Can you work these out from the model? Positions are in its coordinate system, mm. A direction names the side the tool comes from. Coordinates: 2 decimals unless noted, no trailing zeros. Order: outer loops, then holes, each group sorted by start corner. A loop starts at its lowest first (then second) coordinate and runs counter-clockwise, first axis right, second up. Notation, with made-up numbers: (-5.5, 64.5) - (50.5, 64.5) arc R22 ccw to (50.5, 97.5) - close; hole circle Ø3 at (27, -5.75). An arc over 180 degrees is marked (long way). Return JSON: item names as keys, results as strings. Group by question number.
1) Which directions (+Z, -Z, +X, -X, +Y, -Y) give clear straight access to the entire face, cutting with the end or side of a thin tool? Please do faces 4 (the face through (12, -32, 11.049)), 5 (the face through (45, -13.005, 9)), 6 (the face through (16.002, -6, 18)).
2) Imagine slicing it at B-B (z = 23.5). Write out the boundary of the cut face in (x, y) (3 decimals).
3) Imagine slicing it at A-A (y = -6). Write out the boundary of the cut face in (x, z) (3 decimals), and give its area (3 significant figures).
4) Imagine slicing it at C-C (x = 6). Write out the boundary of the cut face in (y, z).
5) For pin 1 Ø5 at (x, z) = (33.5, 19.5) entering from +Y; pin 2 Ø4.5 at (x, y) = (7, -34) entering from +Z; pin 3 Ø18.5 at (y, z) = (-25.5, 5.5) entering from +X, each with a flat end and sliding along its axis, tell me the tip position at first contact or that it passes through.
6) If we mould it in two halves opening along X, with no side actions, what happens to faces 1 (the face through (48, 0, 18)), 2 (the face through (0, -14, 18)), 3 (the face through (28, -11.989, 18))? For each: pulls with the +X half, pulls with the -X half, needs draft (parallel to the pull), parting line crosses it, or undercut.
7) Imagine slicing it at D-D (y = -34.5). Write out the boundary of the cut face in (x, z).
8) If I drill on line 1 along X through (y, z) = (-7.5, 18) (3 decimals); line 2 along X through (y, z) = (-33.5, 25.5); line 3 along X through (y, z) = (-29.5, 7), over which ranges is the centre line in solid material (lowest first)?
```python
from build123d import *

# Parameters (mm, degrees)
F1_DEPTH = 35.9918
F2_W     = 24.9682
F2_H     = 8.9916
F3_DEPTH = 24.9428
F4_W     = 20.8534
F4_H     = 16.9418
F5_DEPTH = 24.003


with BuildPart() as f1:
    # F0 (on Top) → F1 (new body)
    with BuildSketch(Plane.XY):
        Polygon((16.002, 0), (0, 0), (0, -37.0078), (56.007, -37.0078), (56.007, 0), (40.005, 0), (40.005, -11.9888), (16.002, -11.9888), align=None)
    extrude(amount=F1_DEPTH)

    # F2 (on face) → F3 (cut)
    with BuildSketch(Plane.XY.offset(35.9918)):
        with Locations((12.4841, -32.512)):
            Rectangle(F2_W, F2_H)
    extrude(amount=-F3_DEPTH, mode=Mode.SUBTRACT)

    # F4 (on face) → F5 (cut)
    with BuildSketch(Plane.XZ.offset(37.0078)):
        with Locations((45.5803, 8.4709)):
            Rectangle(F4_W, F4_H)
    extrude(amount=-F5_DEPTH, mode=Mode.SUBTRACT)


solid = f1.part
```
Calculated:
{
 "1": {"face 4": "+Z, -X, -Y", "face 5": "-Z, +X, -Y", "face 6": "+Z, -Z, +Y"},
 "2": {"outline": "(0, -28.016) - (24.968, -28.016) - (24.968, -37.008) - (56.007, -37.008) - (56.007, 0) - (40.005, 0) - (40.005, -11.989) - (16.002, -11.989) - (16.002, 0) - (0, 0) - close"},
 "3": {"outline": "(0, 0) - (16.002, 0) - (16.002, 35.992) - (0, 35.992) - close; (40.005, 0) - (56.007, 0) - (56.007, 35.992) - (40.005, 35.992) - close", "area": "1,150 mm2"},
 "4": {"outline": "(-37.01, 0) - (0, 0) - (0, 35.99) - (-28.02, 35.99) - (-28.02, 11.05) - (-37.01, 11.05) - close"},
 "5": {"pin 1": "y = -11.99", "pin 2": "z = 11.05", "pin 3": "x = 35.15"},
 "6": {"face 1": "needs draft", "face 2": "pulls with the -X half", "face 3": "undercut"},
 "7": {"outline": "(0, 0) - (35.15, 0) - (35.15, 16.94) - (56.01, 16.94) - (56.01, 35.99) - (24.97, 35.99) - (24.97, 11.05) - (0, 11.05) - close"},
 "8": {"line 1": "0 to 16.002, 40.005 to 56.007", "line 2": "24.97 to 56.01", "line 3": "0 to 35.15"}
}
